Check sheet for the drawn part. Datum: minimum x, y, z corner. Units: mm. A direction names the side the tool comes from. Coordinates: 2 decimals unless noted, no trailing zeros. Loops run counter-clockwise (first coordinate to the right, second up) from the corner with the lowest first, then second, coordinate; pieces in that order, holes last. Notation, with made-up numbers: M 70.5,-16.75 L 115.5,-16.75 A23 ccw 115.5,0.25 Z; hole C 87,-16 d1. An arc over 180 degrees is marked long. Answer in a Markdown table with one row per item. Add a question column.
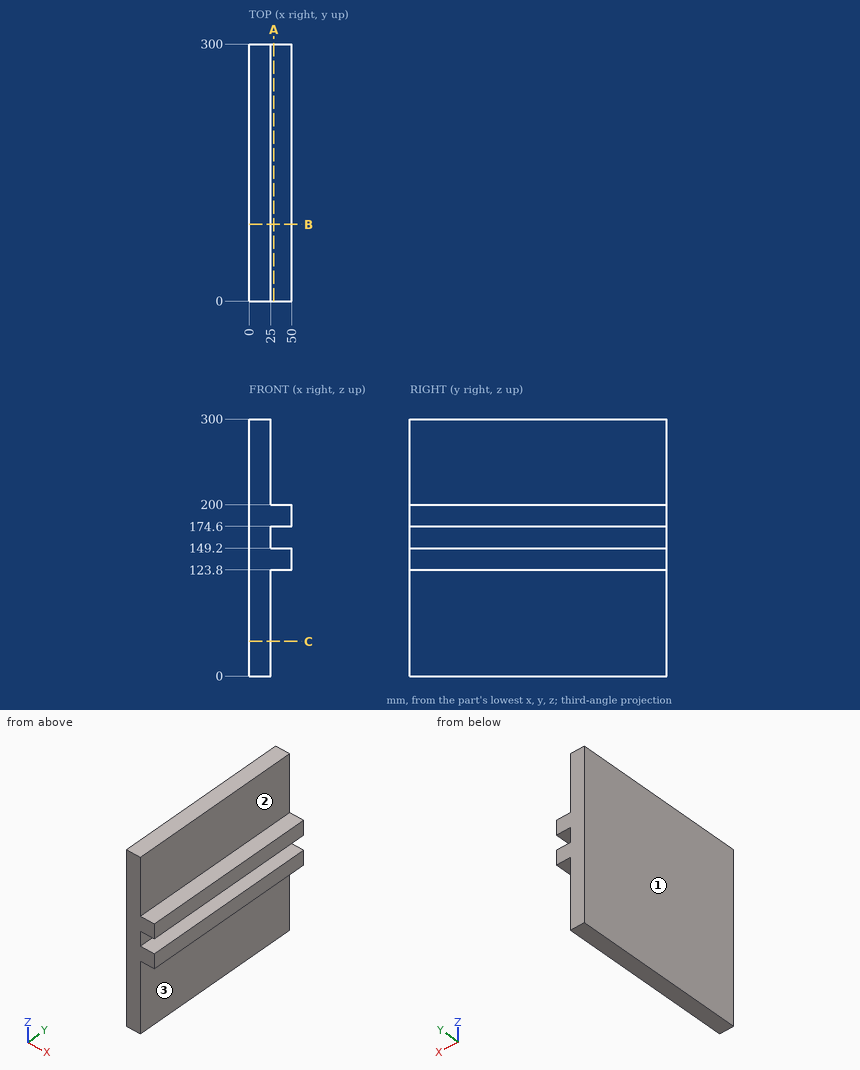
Q1. Access from +Z, -Z, +X, -X, +Y, -Y to the whole of each face (thin tool, end or side, straight path). Record for the marked faces 1, 2 and 3.
Q2. Cross-section at A-A (x = 29). Record the cut outline in (y, z), plus the area to 3 significant figures.
Q3. Cross-section at B-B (y = 89.5). Record the cut outline in (x, z).
Q4. Go/stop test with flat-tipped pins: pin 1 (7.5 mm diameter, centred on x = 35, y = 109.5, fed in from +Z); pin 2 (3 mm diameter, centred on y = 269, z = 216.5, fed in from +X); pin 3 (12.5 mm diameter, centred on x = 38, y = 143.5, fed in from -Z). Record where each tip stops, or that it passes through.
Q5. Thickness scan on L1, parallel to Z at x = 38, y = 106; L2, parallel to X at y = 237, z = 56.5. Record the ranges inside material, lowest first.
Q6. Cross-section at C-C (z = 40.5). Record the cut outline in (x, y).
Answer key:
| question | item | result |
|---|---|---|
| 1 | face 1 | +Z, -Z, -X, +Y, -Y |
| 1 | face 2 | +Z, +X, +Y, -Y |
| 1 | face 3 | -Z, +X, +Y, -Y |
| 2 | outline | M 0,123.8 L 300,123.8 L 300,149.2 L 0,149.2 Z; M 0,174.6 L 300,174.6 L 300,200 L 0,200 Z |
| 2 | area | 15,200 mm^2 |
| 3 | outline | M 0,0 L 25,0 L 25,123.8 L 50,123.8 L 50,149.2 L 25,149.2 L 25,174.6 L 50,174.6 L 50,200 L 25,200 L 25,300 L 0,300 Z |
| 4 | pin 1 | z = 200 |
| 4 | pin 2 | x = 25 |
| 4 | pin 3 | z = 123.8 |
| 5 | L1 | 123.8 to 149.2, 174.6 to 200 |
| 5 | L2 | 0 to 25 |
| 6 | outline | M 0,0 L 25,0 L 25,300 L 0,300 Z |
